```python
from build123d import *

# Parameters (mm, degrees)
SKETCH1_R           = 1.75
BOSS_EXTRUDE1_DEPTH = 53.62
SKETCH3_R           = 0.75
CUT_EXTRUDE1_DEPTH  = 10
SKETCH4_R           = 2.25
BOSS_EXTRUDE2_DEPTH = 7.62


with BuildPart() as part:
    # Sketch1 → Boss-Extrude1 (new body)
    with BuildSketch(Plane.XY):
        with Locations((5.826393973, 0)):
            Circle(SKETCH1_R)
    extrude(amount=BOSS_EXTRUDE1_DEPTH)

    # Sketch3 → Cut-Extrude1 (cut)
    with BuildSketch(Plane.XY.offset(53.62)):
        with Locations((5.826393973, 0)):
            Circle(SKETCH3_R)
    extrude(amount=-CUT_EXTRUDE1_DEPTH, mode=Mode.SUBTRACT)

    # Sketch4 → Boss-Extrude2 (add)
    with BuildSketch(Plane(origin=(0, 0, 0), x_dir=(-1, 0, 0), z_dir=(0, 0, -1))):
        with Locations((-5.826393973, 0)):
            Circle(SKETCH4_R)
    extrude(amount=-BOSS_EXTRUDE2_DEPTH)


solid = part.part
```
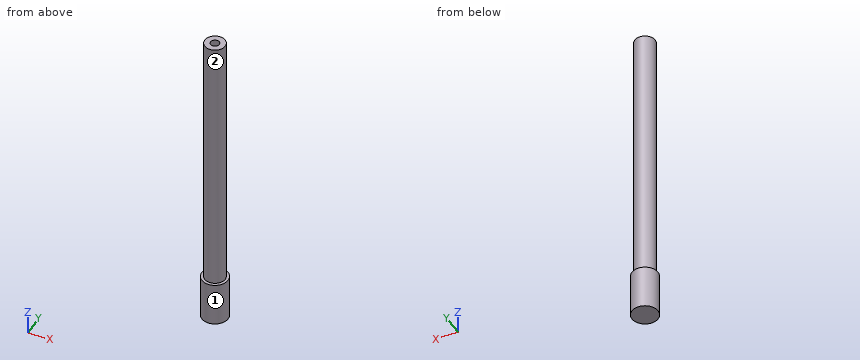
Work out the finished part from the listing and answer in its coordinate system (mm). Face numbers are marked on the shaded views. A direction names the side the tool comes from. Give positions to 0.01 mm unless a question says otherwise; leave off trailing zeros. Loops run counter-clockwise (first coordinate to the right, second up) from the corner with the lowest first, then second, coordinate; pieces in that order, holes last. Notation, with made-up numbers: M -13,1 L 43,1 A14 cw 43,8 Z; hole C 71,23 d9. An arc over 180 degrees is marked long. One line per item, written item: value. Start each with the question number.
1. Find the intervals of material crossed by probe 1 along Y at (x, z) = (5.7, 43.5); probe 2 along Y at (x, z) = (5.85, 44); probe 3 along Z at (x, y) = (4, -1), in increasing order.
2. This flat-tipped pin is pushed along its axis until it touches: P1, Ø1.4, axis at x = 5.83, y = 0, coming from the +Z side. Where does it stop, or does it pass through?
3. Which of the six approach directions +Z, -Z, +X, -X, +Y, -Y give full straight-line access (tool end or side, diameter ignored) to the marked faces 1 and 2?
4. Find section C-C (z = 5.5). Give the vertices of the cut face in (x, y), and give its area (3 significant figures).
5. Find section A-A (y = 0). Give the vertices of the cut face in (x, z), and give its area (3 significant figures).
6. Find section B-B (z = 42). Give the vertices of the cut face in (x, y), and give its area (3 significant figures).
Reported:
1. probe 1: y = -1.75 to 1.75
1. probe 2: y = -1.75 to -0.75, 0.75 to 1.75
1. probe 3: z = 0 to 7.62
2. P1: stops at z = 43.62
3. face 1: +Z, -Z
3. face 2: +Z
4. outline: C 5.83,0 d4.5
4. area: 15.9 mm²
5. outline: M 3.58,0 L 8.08,0 L 8.08,7.62 L 7.58,7.62 L 7.58,53.62 L 6.58,53.62 L 6.58,43.62 L 5.08,43.62 L 5.08,53.62 L 4.08,53.62 L 4.08,7.62 L 3.58,7.62 Z
5. area: 180 mm²
6. outline: C 5.83,0 d3.5
6. area: 9.62 mm²
